Build history of the part. All positions in model axes, mm. Face numbers are marked on the shaded views. A direction names the side the tool comes from. Round coordinates to 2 decimals unless told otherwise and drop trailing zeros. Write each loop counter-clockwise with the first axis right and the second up, starting at its lowest first coordinate (ties: lowest second). Pieces come first, ordered by that corner, then holes.
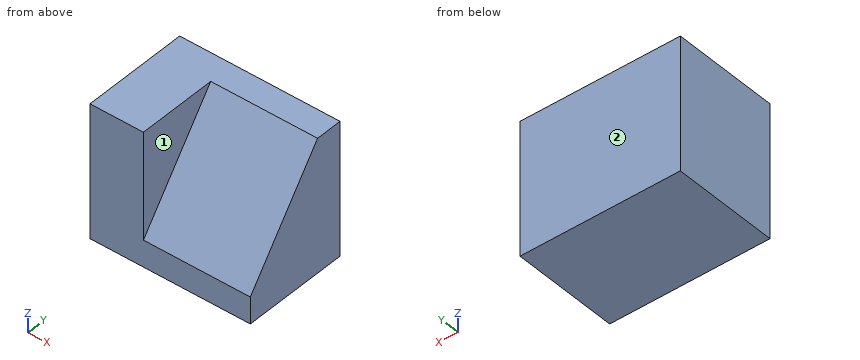
from build123d import *

# Parameters (mm, degrees)
F1_DEPTH = 38.1
F3_DEPTH = 25.4


with BuildPart() as f1:
    # F0 (on Right) → F1 (new body)
    with BuildSketch(Plane.YZ):
        Polygon((-22.806338, 0), (0, 0), (2.593662, 0), (2.593662, 31.75), (-22.806338, 31.75), align=None)
    extrude(amount=F1_DEPTH)

    # F2 (on face) → F3 (cut)
    with BuildSketch(Plane.YZ.offset(38.1)):
        Polygon((-3.756338, 31.75), (-22.806338, 31.75), (-22.806338, 6.35), align=None)
    extrude(amount=-F3_DEPTH, mode=Mode.SUBTRACT)


solid = f1.part
1) Slice it at A-A (x = 21). Write the cut outline in (y, z), plus the area to 3 significant figures.
Results:
outline: (-22.81, 0) - (2.59, 0) - (2.59, 31.75) - (-3.76, 31.75) - (-22.81, 6.35) - close
area: 565 mm2
2) Which spindle directions (+Z, -Z, +X, -X, +Y, -Y) get a long thin tool onto all of the face, cutting with end or side? Do the marked faces 1 and 2. Say none if no direction does.
Results:
face 1: +Z, +X, -Y
face 2: +Z, -Z, +X, -X, +Y
3) Slice it at B-B (y = -9.25). Write the cut outline in (x, z).
Results:
outline: (0, 0) - (38.1, 0) - (38.1, 24.43) - (12.7, 24.43) - (12.7, 31.75) - (0, 31.75) - close
4) Wall check: L1, parallel to X at y = -6.75, z = 30; L2, parallel to Z at x = 31, y = -8.5; L3, parallel to Z at x = 34.5, y = -15.25. Give the ranges that are in metal, low to high.
Results:
L1: x = 0 to 12.7
L2: z = 0 to 25.43
L3: z = 0 to 16.43
5) Slice it at C-C (z = 10.5). Write the cut outline in (x, y), plus the area to 3 significant figures.
Results:
outline: (0, -22.81) - (12.7, -22.81) - (12.7, -19.69) - (38.1, -19.69) - (38.1, 2.59) - (0, 2.59) - close
area: 889 mm2
6) Pin check, flat tips, straight feed: pin 1 Ø1 at (x, y) = (31, -14.5) entering from +Z; pin 2 Ø1 at (x, z) = (29.5, 14) entering from -Y. Stop position of each tip, or through.
Results:
pin 1: stops at z = 18.09
pin 2: stops at y = -17.44
